Design review of the part built by this model. Coordinates are the model's own, in mm. Face numbers are marked on the shaded views. A direction names the side the tool comes from. Give positions to 0.01 mm unless a question says otherwise; leave off trailing zeros. Loops run counter-clockwise (first coordinate to the right, second up) from the corner with the lowest first, then second, coordinate; pieces in that order, holes last. Notation, with made-up numbers: (12.5, 53) -> (61.5, 53) arc R21 ccw to (61.5, 57) -> close; hole circle Ø2 at (-0.5, 13). An arc over 180 degrees is marked (long way). Use a Markdown table: item, result. Add a question column.
1. For pin 1 Ø6.5 at (y, z) = (29.5, 9) entering from +X; pin 2 Ø1 at (x, z) = (-24, 17) entering from +Y; pin 3 Ø4 at (x, z) = (-2.5, 10) entering from +Y; pin 4 Ø3 at (x, z) = (19, 4) entering from +Y, all flat-tipped, find the tip position at first contact; note any pin that passes through.
2. Draft analysis for pull direction X (two halves, no side actions). For the marked faces 4, 5, 6 and 7, state which applies: pulls with the +X half, pulls with the -X half, needs draft (parallel to the pull), parting line crosses it, or undercut.
3. Add section C-C (z = 10). Count the separate pieces of the cut face and the enclosed holes in it, and give its area (3 significant figures).
4. Add section A-A (x = -76.5). State the section outline as (y, z) points.
5. Add section B-B (y = 15.5). State the section outline as (x, z) points.
6. Add section D-D (x = -47.5). State the section outline as (y, z) points, and give its area (3 significant figures).
7. For the marked faces 1, 2 and 3, list the 3-axis set-ups (+Z, -Z, +X, -X, +Y, -Y) from which the entire face can be reached by the end or side of a thin tool; tool diameter is ignored.
8. To check wall thickness, follow line 1 (X direction, y = 10.45, z = 10); line 2 (X direction, y = 13.5, z = 3.75); line 3 (Z direction, x = -2.5, y = 7.6). State the ranges of each line that lie inside material, in increasing order.
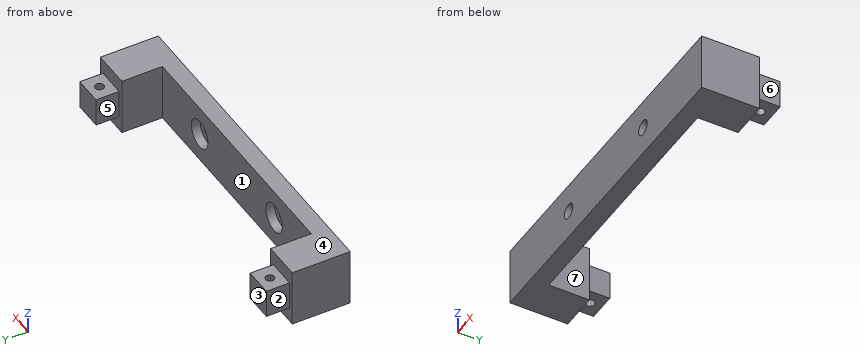
```python
from build123d import *

# Parameters (mm, degrees)
SKETCH_1_W           = 40
SKETCH_1_H           = 20
EXTRUDE_1_DEPTH      = 6
SKETCH_5_W           = 7
SKETCH_5_H           = 20
CUT_EXTRUDE_3_DEPTH  = 6
SKETCH_6_W           = 13
SKETCH_6_H           = 20
EXTRUDE_2_DEPTH      = 20
EXTRUDE_3_DEPTH      = 8
CUT_EXTRUDE_4_DEPTH  = 10
EXTRUDE_4_DEPTH      = 20
EXTRUDE_5_DEPTH      = 8
CUT_EXTRUDE_5_DEPTH  = 10
CUT_EXTRUDE_6_DEPTH  = 3
SKETCH_16_R          = 2.6
CUT_EXTRUDE_7_DEPTH  = 3
CUT_EXTRUDE_8_DEPTH  = 20
SKETCH_19_W          = 90
SKETCH_19_H          = 6
EXTRUDE_6_DEPTH      = 20
CUT_EXTRUDE_9_DEPTH  = 20
SKETCH_21_R          = 5
CUT_EXTRUDE_10_DEPTH = 3


with BuildPart() as part:
    # Sketch 1 → Extrude 1 (new body)
    with BuildSketch(Plane(origin=(0, 0, 0), x_dir=(1, 0, 0), z_dir=(0, 1, 0))):
        with Locations((20, -10)):
            Rectangle(SKETCH_1_W, SKETCH_1_H)
    extrude(amount=EXTRUDE_1_DEPTH)

    # Sketch 5 → Cut-Extrude 3 (cut)
    with BuildSketch(Plane(origin=(0, 6, 0), x_dir=(1, 0, 0), z_dir=(0, 1, 0))):
        with Locations((36.5, -10)):
            Rectangle(SKETCH_5_W, SKETCH_5_H)
    extrude(amount=-CUT_EXTRUDE_3_DEPTH, mode=Mode.SUBTRACT)

    # Sketch 6 → Extrude 2 (add)
    # profile 1 of 3: a face of its own
    with BuildSketch(Plane(origin=(0, 6, 0), x_dir=(1, 0, 0), z_dir=(0, 1, 0))):
        with Locations((26.5, -10)):
            Rectangle(SKETCH_6_W, SKETCH_6_H)
        Polygon((31.5, -5), (31.5, -10), (31.5, -15), (21.5, -15), (21.5, -10), (21.5, -5), align=None, mode=Mode.SUBTRACT)
    # profile 2 of 3: a face of its own
    with BuildSketch(Plane(origin=(0, 6, 0), x_dir=(1, 0, 0), z_dir=(0, 1, 0))):
        Polygon((21.5, -10), (26.5, -10), (31.5, -10), (31.5, -5), (21.5, -5), align=None)
    # profile 3 of 3: a face of its own
    with BuildSketch(Plane(origin=(0, 6, 0), x_dir=(1, 0, 0), z_dir=(0, 1, 0))):
        Polygon((31.5, -10), (26.5, -10), (21.5, -10), (21.5, -15), (31.5, -15), align=None)
    extrude(amount=EXTRUDE_2_DEPTH)

    # Sketch 8 → Extrude 3 (add)
    with BuildSketch(Plane(origin=(0, 26, 0), x_dir=(1, 0, 0), z_dir=(0, 1, 0))):
        Polygon((31.4, -5.1), (23.315, -5.1), (26.5, -10), (31.4, -10), align=None)
        Polygon((26.5, -10), (23.315, -5.1), (21.6, -5.1), (21.6, -10), align=None)
        Polygon((29.685, -14.9), (26.5, -10), (21.6, -10), (21.6, -14.9), align=None)
        Polygon((31.4, -10), (26.5, -10), (29.685, -14.9), (31.4, -14.9), align=None)
    extrude(amount=EXTRUDE_3_DEPTH)

    # Sketch 9 → Cut-Extrude 4 (cut)
    with BuildSketch(Plane.XY.offset(14.9)):
        with BuildLine():
            ThreePointArc((28, 30), (27.560660172, 31.060660172), (26.5, 31.5))
            Line((26.5, 31.5), (26.5, 28.5))
            ThreePointArc((26.5, 28.5), (27.560660172, 28.939339828), (28, 30))
        make_face()
        with BuildLine():
            Line((26.5, 28.5), (26.5, 31.5))
            ThreePointArc((26.5, 31.5), (25, 30), (26.5, 28.5))
        make_face()
    extrude(amount=-CUT_EXTRUDE_4_DEPTH, mode=Mode.SUBTRACT)

    # Sketch 10 → Extrude 4 (add)
    with BuildSketch(Plane.XY.offset(20)):
        Polygon((0, 0), (0, 6), (-70, 6), (-70, 26), (-83, 26), (-83, 0), align=None)
    extrude(amount=-EXTRUDE_4_DEPTH)

    # Sketch 12 → Extrude 5 (add)
    with BuildSketch(Plane(origin=(0, 26, 0), x_dir=(1, 0, 0), z_dir=(0, 1, 0))):
        Polygon((-71.6, -5.1), (-79.685, -5.1), (-76.5, -10), (-71.6, -10), align=None)
        Polygon((-76.5, -10), (-79.685, -5.1), (-81.4, -5.1), (-81.4, -10), align=None)
        Polygon((-73.315, -14.9), (-76.5, -10), (-81.4, -10), (-81.4, -14.9), align=None)
        Polygon((-71.6, -10), (-76.5, -10), (-73.315, -14.9), (-71.6, -14.9), align=None)
    extrude(amount=EXTRUDE_5_DEPTH)

    # Sketch 13 → Cut-Extrude 5 (cut)
    with BuildSketch(Plane.XY.offset(14.9)):
        with BuildLine():
            ThreePointArc((-75, 30), (-75.996506058, 31.412973407), (-77.6619918, 30.948564735))
            Line((-77.6619918, 30.948564735), (-75.3380082, 29.051435265))
            ThreePointArc((-75.3380082, 29.051435265), (-75.087026593, 29.496506058), (-75, 30))
        make_face()
        with BuildLine():
            Line((-75.3380082, 29.051435265), (-77.6619918, 30.948564735))
            ThreePointArc((-77.6619918, 30.948564735), (-77.448564735, 28.8380082), (-75.3380082, 29.051435265))
        make_face()
    extrude(amount=-CUT_EXTRUDE_5_DEPTH, mode=Mode.SUBTRACT)

    # Sketch 15 → Cut-Extrude 6 (cut)
    with BuildSketch(Plane(origin=(0, 6, 0), x_dir=(1, 0, 0), z_dir=(0, 1, 0))):
        with BuildLine():
            ThreePointArc((-52.5, -10), (-47.5, -15), (-42.5, -10))
            Line((-42.5, -10), (-52.5, -10))
        make_face()
        with BuildLine():
            Line((-52.5, -10), (-42.5, -10))
            ThreePointArc((-42.5, -10), (-47.5, -5), (-52.5, -10))
        make_face()
        with BuildLine():
            ThreePointArc((2.5, -10), (-2.5, -5), (-7.5, -10))
            Line((-7.5, -10), (2.5, -10))
        make_face()
        with BuildLine():
            Line((2.5, -10), (-7.5, -10))
            ThreePointArc((-7.5, -10), (-2.5, -15), (2.5, -10))
        make_face()
    extrude(amount=-CUT_EXTRUDE_6_DEPTH, mode=Mode.SUBTRACT)

    # Sketch 16 → Cut-Extrude 7 (cut)
    with BuildSketch(Plane(origin=(0, 3, 0), x_dir=(1, 0, 0), z_dir=(0, 1, 0))):
        with Locations(Location((-47.5, -10, 0), (0, 0, 270))):
            Circle(SKETCH_16_R)
        with Locations(Location((-2.5, -10, 0), (0, 0, 270))):
            Circle(SKETCH_16_R)
    extrude(amount=-CUT_EXTRUDE_7_DEPTH, mode=Mode.SUBTRACT)

    # Sketch 18 → Cut-Extrude 8 (cut)
    with BuildSketch(Plane(origin=(0, 0, 0), x_dir=(-1, 0, 0), z_dir=(0, 0, -1))):
        Polygon((-20, 6), (-33, 6), (-33, 0), (83, 0), (83, 6), (70, 6), align=None)
    extrude(amount=-CUT_EXTRUDE_8_DEPTH, mode=Mode.SUBTRACT)


with BuildPart() as cut_extrude_8_piece_1:
    # of the separate pieces the step leaves, piece 1, a body of its own (cut_extrude_8_pieces)
    add(part.part.solids().sort_by_distance((-70, 6, 0))[0])



with BuildPart() as cut_extrude_8_piece_2:
    # of the separate pieces the step leaves, piece 2, a body of its own (cut_extrude_8_pieces)
    add(part.part.solids().sort_by_distance((33, 26, 0))[0])


with BuildPart() as cut_extrude_8_piece_1_1:
    add(cut_extrude_8_piece_1.part)

    add(cut_extrude_8_piece_2.part)  # Extrude 6 merges Cut-Extrude 8 piece 2
    # Sketch 19 → Extrude 6 (add)
    with BuildSketch(Plane(origin=(0, 0, 0), x_dir=(-1, 0, 0), z_dir=(0, 0, -1))):
        with Locations((25, 9)):
            Rectangle(SKETCH_19_W, SKETCH_19_H)
    extrude(amount=-EXTRUDE_6_DEPTH)

    # Sketch 20 → Cut-Extrude 9 (cut)
    with BuildSketch(Plane(origin=(0, 12, 0), x_dir=(1, 0, 0), z_dir=(0, 1, 0))):
        with BuildLine():
            ThreePointArc((-50.1, -10), (-47.5, -12.6), (-44.9, -10))
            Line((-44.9, -10), (-50.1, -10))
        make_face()
        with BuildLine():
            Line((-50.1, -10), (-44.9, -10))
            ThreePointArc((-44.9, -10), (-47.5, -7.4), (-50.1, -10))
        make_face()
        with BuildLine():
            ThreePointArc((0.1, -10), (-2.5, -7.4), (-5.1, -10))
            Line((-5.1, -10), (0.1, -10))
        make_face()
        with BuildLine():
            Line((0.1, -10), (-5.1, -10))
            ThreePointArc((-5.1, -10), (-2.5, -12.6), (0.1, -10))
        make_face()
    extrude(amount=-CUT_EXTRUDE_9_DEPTH, mode=Mode.SUBTRACT)

    # Sketch 21 → Cut-Extrude 10 (cut)
    with BuildSketch(Plane(origin=(0, 12, 0), x_dir=(1, 0, 0), z_dir=(0, 1, 0))):
        with Locations(Location((-47.5, -10, 0), (0, 0, 270))):
            Circle(SKETCH_21_R)
        with Locations(Location((-2.5, -10, 0), (0, 0, 270))):
            Circle(SKETCH_21_R)
    extrude(amount=-CUT_EXTRUDE_10_DEPTH, mode=Mode.SUBTRACT)


solid = cut_extrude_8_piece_1_1.part
```
Taken from the geometry:
| question | item | result |
|---|---|---|
| 1 | pin 1 | stops at x = 31.4 |
| 1 | pin 2 | stops at y = 12 |
| 1 | pin 3 | passes through |
| 1 | pin 4 | stops at y = 26 |
| 2 | face 4 | needs draft |
| 2 | face 5 | undercut |
| 2 | face 6 | pulls with the +X half |
| 2 | face 7 | undercut |
| 3 | separate pieces | 3 |
| 3 | enclosed holes | 2 |
| 3 | area | 1,110 mm^2 |
| 4 | outline | (6, 0) -> (26, 0) -> (26, 5.1) -> (28.5, 5.1) -> (28.5, 14.9) -> (26, 14.9) -> (26, 20) -> (6, 20) -> close; (31.5, 5.1) -> (34, 5.1) -> (34, 14.9) -> (31.5, 14.9) -> close |
| 5 | outline | (-83, 0) -> (-70, 0) -> (-70, 20) -> (-83, 20) -> close; (20, 0) -> (33, 0) -> (33, 20) -> (20, 20) -> close |
| 6 | outline | (6, 0) -> (12, 0) -> (12, 5) -> (9, 5) -> (9, 7.4) -> (6, 7.4) -> close; (6, 12.6) -> (9, 12.6) -> (9, 15) -> (12, 15) -> (12, 20) -> (6, 20) -> close |
| 6 | area | 74.4 mm^2 |
| 7 | face 1 | +Z, -Z, +Y |
| 7 | face 2 | +Z, -Z, -X, +Y |
| 7 | face 3 | +Z, -Z, +X, -X, +Y |
| 8 | line 1 | x = -83 to -52.5, -42.5 to -7.5, 2.5 to 33 |
| 8 | line 2 | x = -83 to -70, 20 to 33 |
| 8 | line 3 | z = 0 to 7.4, 12.6 to 20 |
